Could you check a few things on this drawing? It's one solid part, dimensions in mm from its lowest x, y, z. A direction names the side the tool comes from. Coordinates: 2 decimals unless noted, no trailing zeros. Order: outer loops, then holes, each group sorted by start corner. A loop starts at its lowest first (then second) coordinate and runs counter-clockwise, first axis right, second up. Notation, with made-up numbers: (-35.75, 48) -> (2.25, 48) arc R14 ccw to (2.25, 61) -> close; hole circle Ø5 at (81, 51.5). An arc over 180 degrees is marked (long way). Answer as CSV lines item,"result".
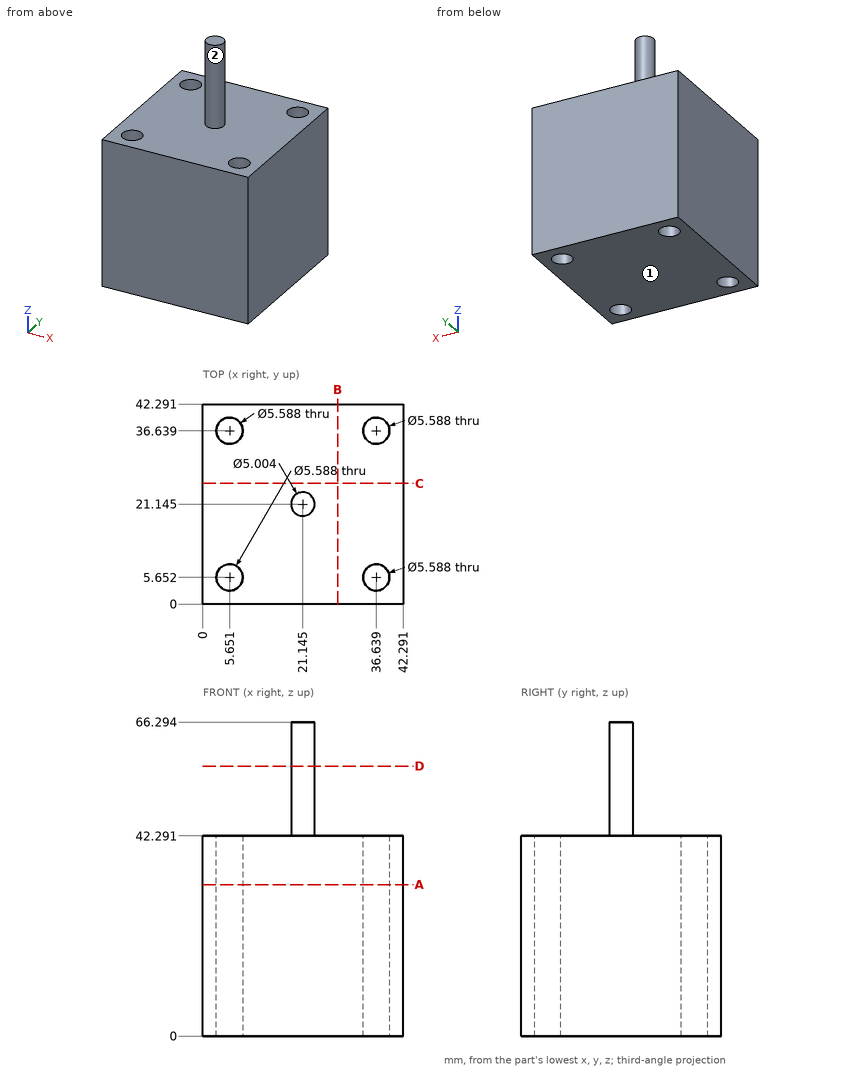
Q1. For P1, Ø8, axis at y = 30.5, z = 53, coming from the +X side; P2, Ø6.5, axis at x = 5.65, y = 36.64, coming from the +Z side, each with a flat end and sliding along its axis, tell me the tip position at first contact or that it passes through.
Solution:
P1,"through"
P2,"z = 42.29"
Q2. Imagine slicing it at D-D (z = 57). List the corners of the cut face in (x, y) for me (1 decimal).
Solution:
outline,"circle Ø5 at (21.1, 21.1)"
Q3. If I drill on line 1 (X direction, y = 6, z = 7); line 2 (Y direction, x = 7.5, z = 18) (1 decimal); line 3 (Z direction, x = 39.5, y = 11), over which ranges is the centre line in solid material (lowest first)?
Solution:
line 1,"0 to 2.88, 8.42 to 33.87, 39.41 to 42.29"
line 2,"0 to 3.6, 7.7 to 34.5, 38.7 to 42.3"
line 3,"0 to 42.29"
Q4. Imagine slicing it at A-A (z = 32). List the corners of the cut face in (x, y) for me (1 decimal).
Solution:
outline,"(0, 0) -> (42.3, 0) -> (42.3, 42.3) -> (0, 42.3) -> close; hole circle Ø5.6 at (5.7, 5.7); hole circle Ø5.6 at (5.7, 36.6); hole circle Ø5.6 at (36.6, 5.7); hole circle Ø5.6 at (36.6, 36.6)"
Q5. Which directions (+Z, -Z, +X, -X, +Y, -Y) give clear straight access to the entire face, cutting with the end or side of a thin tool? Please do the marked faces 1 and 2.
Solution:
face 1,"-Z, +X, -X, +Y, -Y"
face 2,"+Z"
Q6. Imagine slicing it at B-B (x = 28.5). List the corners of the cut face in (y, z) for me.
Solution:
outline,"(0, 0) -> (42.29, 0) -> (42.29, 42.29) -> (0, 42.29) -> close"
